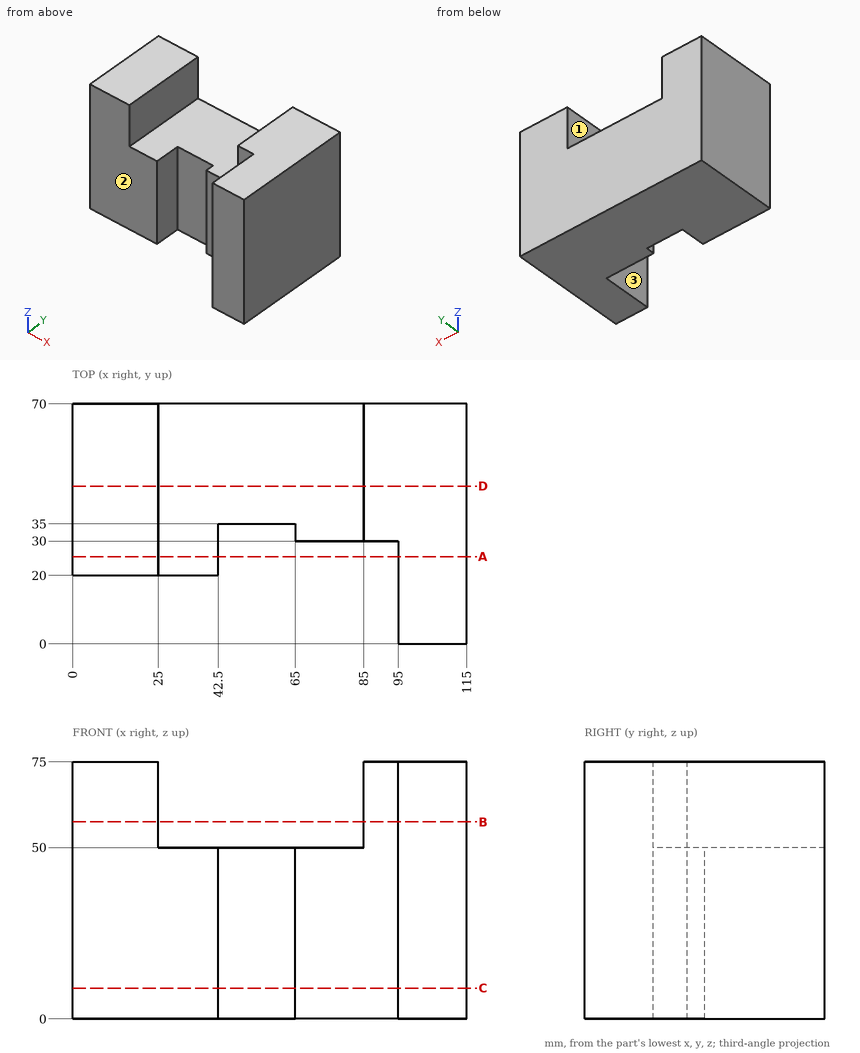
Verification items for this drawing (mm, ordinates from the low corner). A direction names the side the tool comes from. Round coordinates to 2 decimals unless told otherwise and drop trailing zeros. Loops run counter-clockwise (first coordinate to the right, second up) from the corner with the lowest first, then second, coordinate; pieces in that order, holes last. Notation, with made-up numbers: (-1, -27) - (6, -27) arc R12 cw to (6, -16) - close; hole circle Ø3 at (32, 73.5). An arc over 180 degrees is marked (long way). Answer as CSV lines item,"result". Start each with the question number.
Item 1: Section check C-C (z = 9). Record the boundary of the cut face in (x, y), and give its area (3 significant figures).
Item 2: Section check B-B (z = 57.5). Record the boundary of the cut face in (x, y).
Item 3: Depth check by flat-ended pin: P1, Ø15, axis at x = 76, z = 48.5, coming from the -Y side; P2, Ø1.5, axis at x = 72.5, y = 60, coming from the +Z side; P3, Ø25, axis at x = 52.5, z = 37, coming from the -Y side. Enter the tip coordinate at first touch or a pass-through.
Item 4: Scan lines: line 1 (Y direction, x = 24, z = 15); line 2 (X direction, y = 57, z = 64); line 3 (Y direction, x = 45, z = 18). Record each from-to range of solid material in increasing order. Write a range as [from, to].
Item 5: Set-up check for the marked faces 1, 2 and 3: record each of +Z, -Z, +X, -X, +Y, -Y from which the full face is reachable in a straight line by a thin tool's end or side.
Item 6: Section check D-D (y = 46). Record the boundary of the cut face in (x, z).
Item 7: Section check A-A (y = 25.5). Record the boundary of the cut face in (x, z).
Report:
1,outline,"(0, 20) - (42.5, 20) - (42.5, 35) - (65, 35) - (65, 30) - (95, 30) - (95, 0) - (115, 0) - (115, 70) - (0, 70) - close"
1,area,"5,510 mm2"
2,outline,"(0, 20) - (25, 20) - (25, 70) - (0, 70) - close; (85, 30) - (95, 30) - (95, 0) - (115, 0) - (115, 70) - (85, 70) - close"
3,P1,"stops at y = 30"
3,P2,"stops at z = 50"
3,P3,"stops at y = 20"
4,line 1,"y = [20, 70]"
4,line 2,"x = [0, 25], [85, 115]"
4,line 3,"y = [35, 70]"
5,face 1,"+Z, +Y, -Y"
5,face 2,"+Z, -Z, -X, -Y"
5,face 3,"+Z, -Z, -Y"
6,outline,"(0, 0) - (115, 0) - (115, 75) - (85, 75) - (85, 50) - (25, 50) - (25, 75) - (0, 75) - close"
7,outline,"(0, 0) - (42.5, 0) - (42.5, 50) - (25, 50) - (25, 75) - (0, 75) - close; (95, 0) - (115, 0) - (115, 75) - (95, 75) - close"
